Can you work these out from the model? Positions are in its coordinate system, mm. Coordinates: 2 decimals unless noted, no trailing zeros. Write each loop counter-clockwise with the first axis right and the second up, starting at its lowest first coordinate (ties: lowest second). Pieces come first, ordered by that corner, then holes. Notation, with made-up numbers: (32.25, -30) -> (82.25, -30) arc R19 cw to (82.25, -3) -> close; hole circle Ø6 at (83, 3). An arc over 180 degrees is marked (long way). Use one line per item in the form item = value.
```python
from build123d import *

# Parameters (mm, degrees)
SKETCH1_W           = 70
SKETCH1_H           = 55
BOSS_EXTRUDE1_DEPTH = 5.5
FILLET1_R           = 4.5


with BuildPart() as part:
    # Sketch1 → Boss-Extrude1 (new, symmetric)
    with BuildSketch(Plane(origin=(0, 0, 0), x_dir=(1, 0, 0), z_dir=(0, 1, 0))):
        Rectangle(SKETCH1_W, SKETCH1_H)
    extrude(amount=BOSS_EXTRUDE1_DEPTH, both=True)

    # Fillet1
    fillet1_edges = [part.edges().sort_by_distance(p)[0] for p in [
        (0, 5.5, 27.5),
        (35, 5.5, 0),
        (0, -5.5, 27.5),
        (0, -5.5, -27.5),
        (35, -5.5, 0),
        (35, 0, 27.5),
        (-35, 0, 27.5),
        (-35, 0, -27.5),
        (35, 0, -27.5),
        (0, 5.5, -27.5),
    ]]
    fillet(fillet1_edges, radius=FILLET1_R)


solid = part.part
```
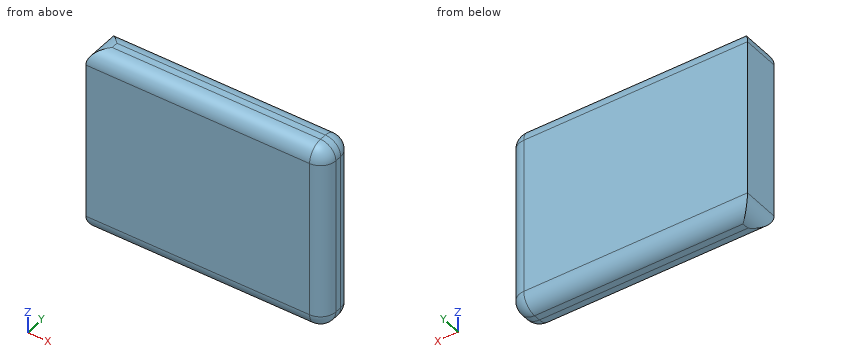
Q1. Will these pins go through, and if not, where does the flat tip stop? pin 1 (4 mm diameter, centred on y = 4, z = 2, fed in from +X); pin 2 (2 mm diameter, centred on x = -5, y = -4, fed in from -Z).
Return value:
pin_1 = 34.89
pin_2 = -27.03
Q2. Suppose I cut it at A-A (x = -25). Write out the boundary of the cut face in (y, z).
Return value:
outline = (-5.5, -23) arc R4.5 ccw to (-1, -27.5) -> (1, -27.5) arc R4.5 ccw to (5.5, -23) -> (5.5, 23) arc R4.5 ccw to (1, 27.5) -> (-1, 27.5) arc R4.5 ccw to (-5.5, 23) -> close
Q3. Suppose I cut it at B-B (y = 4.25). Write out the boundary of the cut face in (x, z).
Return value:
outline = (-35, -23) arc R4.5 ccw to (-33.75, -26.11) -> (30.5, -26.11) arc R3.11 ccw to (33.61, -23) -> (33.61, 23) arc R3.11 ccw to (30.5, 26.11) -> (-33.75, 26.11) arc R4.5 ccw to (-35, 23) -> close
Q4. If I drill on line 1 (X direction, y = -1.25, z = 0); line 2 (Z direction, x = 24.5, y = 1.75); line 3 (Y direction, x = 32.5, z = -10.5), over which ranges is the centre line in solid material (lowest first)? Write a range as from..to.
Return value:
line_1 = -35..34.99
line_2 = -27.44..27.44
line_3 = -5.03..5.03
